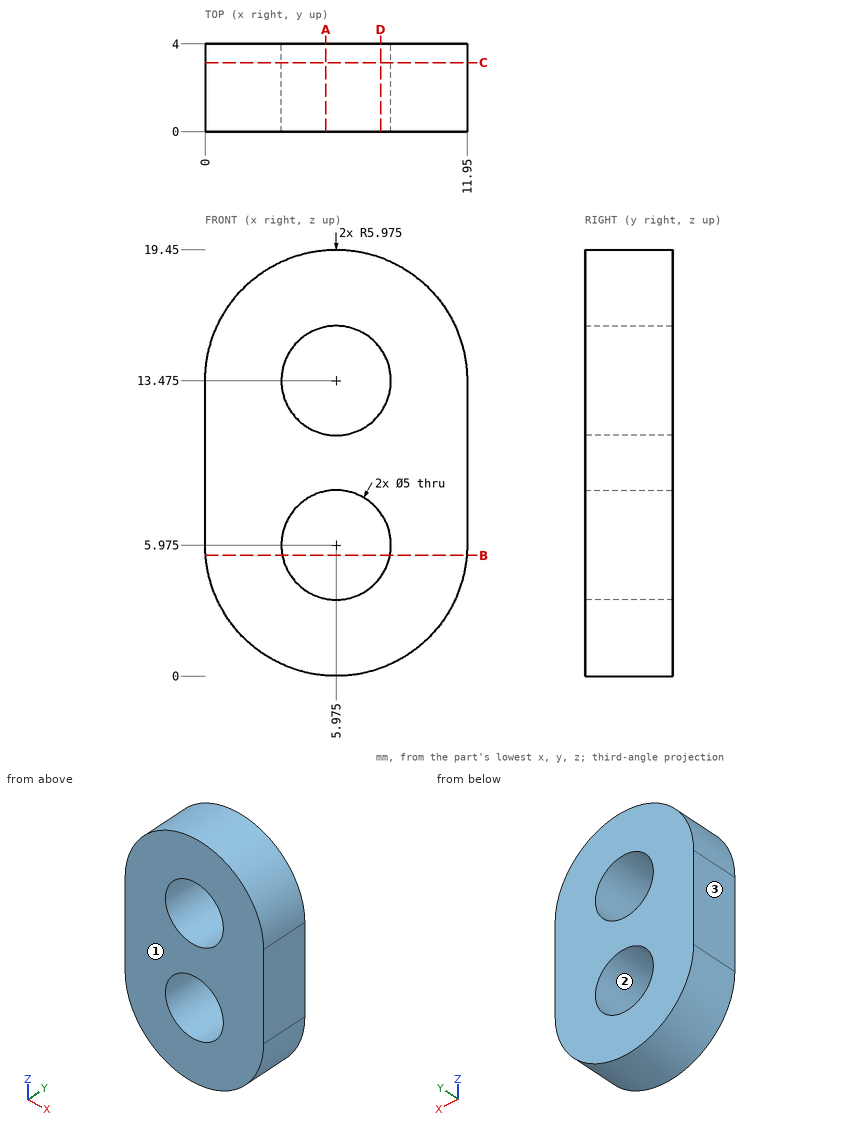
Can you work these out from the drawing? Everything is in mm from the part's minimum corner. Give positions to 0.01 mm unless a question says otherwise; leave off trailing zeros. Order: outer loops, then holes, each group sorted by start corner. A loop starts at its lowest first (then second) coordinate and runs counter-clockwise, first axis right, second up. Notation, with made-up numbers: M 31,17 L 63,17 A22 ccw 63,25 Z; hole C -4.5,67.5 d10. An arc over 180 degrees is marked long. Use a Markdown table: item, result. Add a question column.
Item 1: Suppose I cut it at B-B (z = 5.5). List the corners of the cut face in (x, y) for me.
Item 2: We'd pull the mould along X, two halves only. Please class the marked faces 1, 2 and 3: +X half, -X half, draft (parallel to the pull), parting line (faces both ways), or undercut.
Item 3: Will these pins go through, and if not, where does the flat tip stop? pin 1 (2 mm diameter, centred on x = 1.5, y = 0.5, fed in from -Z); pin 2 (1 mm diameter, centred on y = 3, z = 2, fed in from -X); pin 3 (4.5 mm diameter, centred on x = 5.98, z = 5.98, fed in from -Y).
Item 4: Suppose I cut it at C-C (y = 3.15). List the corners of the cut face in (x, z) for me (3 decimals).
Item 5: Suppose I cut it at D-D (x = 8). List the corners of the cut face in (y, z) for me.
Item 6: Suppose I cut it at A-A (x = 5.5). List the corners of the cut face in (y, z) for me.
Item 7: If I drill on L1, parallel to Z at x = 6, y = 3.6 (3 decimals); L2, parallel to Z at x = 5, y = 1.3; L3, parallel to X at y = 3.7, z = 15.5, over which ranges is the centre line in solid material (lowest first)? Write a range as [from, to].
Answer sheet:
| question | item | result |
|---|---|---|
| 1 | outline | M 0.02,0 L 3.52,0 L 3.52,4 L 0.02,4 Z; M 8.43,0 L 11.93,0 L 11.93,4 L 8.43,4 Z |
| 2 | face 1 | draft |
| 2 | face 2 | undercut |
| 2 | face 3 | -X half |
| 3 | pin 1 | stops at z = 1.11 |
| 3 | pin 2 | stops at x = 1.11 |
| 3 | pin 3 | passes through |
| 4 | outline | M 0,5.975 A5.975 ccw 11.95,5.975 L 11.95,13.475 A5.975 ccw 0,13.475 Z; hole C 5.975,5.975 d5; hole C 5.975,13.475 d5 |
| 5 | outline | M 0,0.35 L 4,0.35 L 4,4.51 L 0,4.51 Z; M 0,7.44 L 4,7.44 L 4,12.01 L 0,12.01 Z; M 0,14.94 L 4,14.94 L 4,19.1 L 0,19.1 Z |
| 6 | outline | M 0,0.02 L 4,0.02 L 4,3.52 L 0,3.52 Z; M 0,8.43 L 4,8.43 L 4,11.02 L 0,11.02 Z; M 0,15.93 L 4,15.93 L 4,19.43 L 0,19.43 Z |
| 7 | L1 | z = [0, 3.475], [8.475, 10.975], [15.975, 19.45] |
| 7 | L2 | z = [0.08, 3.67], [8.28, 11.17], [15.78, 19.37] |
| 7 | L3 | x = [0.35, 4.51], [7.44, 11.6] |
